Could you check a few things on this model? Use its own coordinates, in mm. Give positions to 0.01 mm unless a question says otherwise; leave off trailing zeros. Loops run counter-clockwise (first coordinate to the right, second up) from the corner with the lowest first, then second, coordinate; pieces in that order, holes last. Notation, with made-up numbers: M 18.25,51 L 49.25,51 A23 cw 49.25,73 Z; hole C 82,-4.75 d6. An arc over 180 degrees is marked long. Answer in a Markdown table with one row per item. Add a question column.
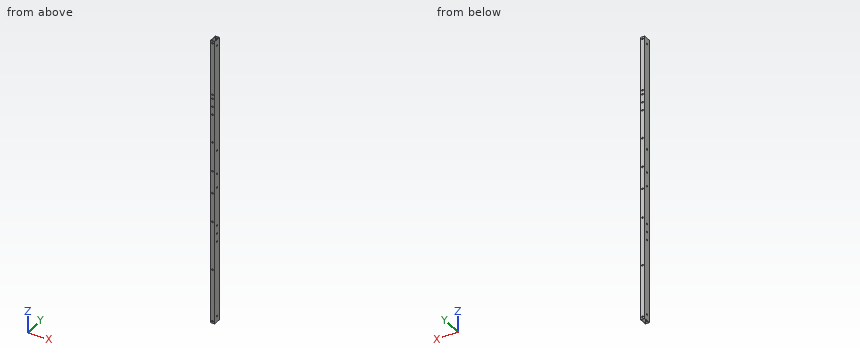
```python
from build123d import *

# Parameters (mm, degrees)
SKETCH_1_W          = 10
SKETCH_1_H          = 20
SKETCH_1_W_2        = 7.6
SKETCH_1_H_2        = 17.6
EXTRUDE_1_DEPTH     = 710
SKETCH_2_R          = 2.15
CUT_EXTRUDE_1_DEPTH = 711.299232718
SKETCH_3_R          = 2.15
CUT_EXTRUDE_2_DEPTH = 711.140831103


with BuildPart() as part:
    # ｽｹｯﾁ1 → 押し出し-薄板1 (new body)
    with BuildSketch(Plane.XY):
        Rectangle(SKETCH_1_W, SKETCH_1_H)
        Rectangle(SKETCH_1_W_2, SKETCH_1_H_2, mode=Mode.SUBTRACT)
    extrude(amount=EXTRUDE_1_DEPTH)

    # ｽｹｯﾁ2 → ｶｯﾄ - 押し出し1 (cut, through all)
    with BuildSketch(Plane(origin=(0, 10, 0), x_dir=(1, 0, 0), z_dir=(0, 1, 0))):
        with Locations(Location((0, -135, 0), (0, 0, 270))):
            Circle(SKETCH_2_R)
        with Locations(Location((0, -5, 0), (0, 0, 270))):
            Circle(SKETCH_2_R)
        with Locations(Location((0, -575, 0), (0, 0, 270))):
            Circle(SKETCH_2_R)
        with Locations(Location((0, -705, 0), (0, 0, 270))):
            Circle(SKETCH_2_R)
        with Locations(Location((0, -255, 0), (0, 0, 270))):
            Circle(SKETCH_2_R)
        with Locations(Location((0, -455, 0), (0, 0, 270))):
            Circle(SKETCH_2_R)
        with Locations(Location((0, -565, 0), (0, 0, 270))):
            Circle(SKETCH_2_R)
        with Locations(Location((0, -525, 0), (0, 0, 270))):
            Circle(SKETCH_2_R)
        with Locations(Location((0, -545, 0), (0, 0, 270))):
            Circle(SKETCH_2_R)
        with Locations(Location((0, -327.5, 0), (0, 0, 270))):
            Circle(SKETCH_2_R)
        with Locations(Location((0, -382.5, 0), (0, 0, 270))):
            Circle(SKETCH_2_R)
    extrude(amount=-CUT_EXTRUDE_1_DEPTH, mode=Mode.SUBTRACT)

    # ｽｹｯﾁ3 → ｶｯﾄ - 押し出し2 (cut, through all)
    with BuildSketch(Plane(origin=(5, 0, 0), x_dir=(0, 0, -1), z_dir=(1, 0, 0))):
        with Locations(Location((-202.5, 0, 0), (0, 0, 90))):
            Circle(SKETCH_3_R)
        with Locations(Location((-222.5, 0, 0), (0, 0, 90))):
            Circle(SKETCH_3_R)
        with Locations(Location((-242.5, 0, 0), (0, 0, 90))):
            Circle(SKETCH_3_R)
        with Locations(Location((-430.5, 0, 0), (0, 0, 90))):
            Circle(SKETCH_3_R)
        with Locations(Location((-14.5, 0, 0), (0, 0, 90))):
            Circle(SKETCH_3_R)
        with Locations(Location((-695.5, 0, 0), (0, 0, 90))):
            Circle(SKETCH_3_R)
        with Locations(Location((-372.5, 0, 0), (0, 0, 90))):
            Circle(SKETCH_3_R)
        with Locations(Location((-337.5, 0, 0), (0, 0, 90))):
            Circle(SKETCH_3_R)
    extrude(amount=-CUT_EXTRUDE_2_DEPTH, mode=Mode.SUBTRACT)


solid = part.part
```
Item 1: Suppose I cut it at B-B (x = 0). Give the number of separate pieces and of enclosed holes in the cut face, then the cut area to 3 significant figures.
Item 2: For P1, Ø5, axis at x = 0, z = 135, coming from the -Y side, with a flat end and sliding along its axis, tell me the tip position at first contact or that it passes through.
Item 3: I need wall thicknesses on L1, parallel to X at y = -8.75, z = 533.5; L2, parallel to Y at x = -0.75, z = 645.5; L3, parallel to Y at x = -4.35, z = 242.5. Which ranges of each line are inside material? Lowest first, please.
Item 4: Suppose I cut it at A-A (z = 420). List the corners of the cut face in (x, y) for me, then the cut area to 3 significant figures.
Values found:
| question | item | result |
|---|---|---|
| 1 | separate pieces | 24 |
| 1 | enclosed holes | 0 |
| 1 | area | 1,590 mm² |
| 2 | P1 | y = -10 |
| 3 | L1 | -5 to -3.8, 3.8 to 5 |
| 3 | L2 | -10 to -8.8, 8.8 to 10 |
| 3 | L3 | -10 to -2.15, 2.15 to 10 |
| 4 | outline | M -5,-10 L 5,-10 L 5,10 L -5,10 Z; hole M -3.8,-8.8 L 3.8,-8.8 L 3.8,8.8 L -3.8,8.8 Z |
| 4 | area | 66.2 mm² |
